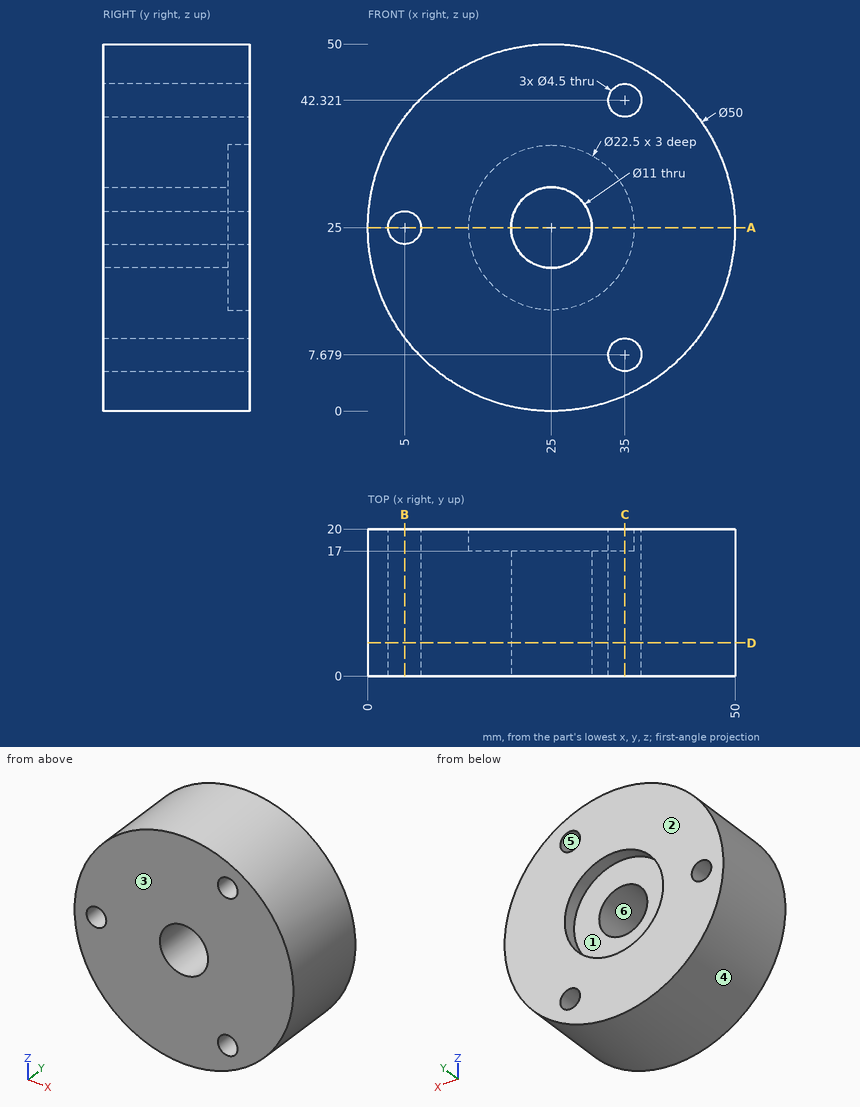
Can you work these out from the drawing? Everything is in mm from the part's minimum corner. A direction names the side the tool comes from. Give positions to 0.01 mm unless a question says otherwise; leave off trailing zeros. Order: outer loops, then holes, each group sorted by start corner. A loop starts at its lowest first (then second) coordinate and runs counter-clockwise, first axis right, second up.
Item 1: If we section it at D-D, the plane y = 4.5: Count the separate pieces of the cut face and the enclosed holes in it, plus the area to 3 significant figures.
Item 2: If we section it at C-C, the plane x = 35: Write out the boundary of the cut face in (y, z).
Item 3: If we section it at B-B, the plane x = 5: Write out the boundary of the cut face in (y, z), plus the area to 3 significant figures.
Item 4: If we mould it in two halves opening along X, with no side actions, what happens to the marked faces 3, 4, 5 and 6? For each: pulls with the +X half, pulls with the -X half, needs draft (parallel to the pull), parting line crosses it, or undercut.
Item 5: For the marked faces 1 and 2, which set-ups out of +Z, -Z, +X, -X, +Y, -Y let a thin tool reach every point of the face, with its end or its side?
Item 6: If we section it at A-A, the plane z = 25: Write out the boundary of the cut face in (x, y).
Item 7: I'm going to push flat-ended pins straight in: pin 1 (6 mm diameter, centred on x = 9.5, y = 17, fed in from -Z); pin 2 (10 mm diameter, centred on y = 4, z = 11.5, fed in from -X); pin 3 (1 mm diameter, centred on x = 37.5, y = 10.5, fed in from +Z). Where does each tip first touch, or does it pass through?
Item 8: I need wall thicknesses on line 1 (X direction, y = 13.5, z = 25); line 2 (X direction, y = 19.25, z = 25); line 3 (Y direction, x = 25.5, z = 18.5). Which ranges of each line are inside material? Lowest first, please.
Values:
1. separate pieces: 1
1. enclosed holes: 4
1. area: 1,820 mm2
2. outline: (0, 2.09) - (20, 2.09) - (20, 5.43) - (0, 5.43) - close; (0, 9.93) - (20, 9.93) - (20, 19.85) - (17, 19.85) - (17, 30.15) - (20, 30.15) - (20, 40.07) - (0, 40.07) - close; (0, 44.57) - (20, 44.57) - (20, 47.91) - (0, 47.91) - close
3. outline: (0, 10) - (20, 10) - (20, 22.75) - (0, 22.75) - close; (0, 27.25) - (20, 27.25) - (20, 40) - (0, 40) - close
3. area: 510 mm2
4. face 3: needs draft
4. face 4: parting line crosses it
4. face 5: undercut
4. face 6: undercut
5. face 1: +Y
5. face 2: +Z, -Z, +X, -X, +Y
6. outline: (0, 0) - (2.75, 0) - (2.75, 20) - (0, 20) - close; (7.25, 0) - (19.5, 0) - (19.5, 17) - (13.75, 17) - (13.75, 20) - (7.25, 20) - close; (30.5, 0) - (50, 0) - (50, 20) - (36.25, 20) - (36.25, 17) - (30.5, 17) - close
7. pin 1: stops at z = 3.35
7. pin 2: stops at x = 1.49
7. pin 3: stops at z = 46.93
8. line 1: x = 0 to 2.75, 7.25 to 19.5, 30.5 to 50
8. line 2: x = 0 to 2.75, 7.25 to 13.75, 36.25 to 50
8. line 3: y = 0 to 17
